from build123d import *

# Parameters (mm, degrees)
F3_D     = 1.1
F5_DEPTH = 11


with BuildPart() as f1:
    # F0 (on Front) → F1 (revolve)
    with BuildSketch(Plane.XZ):
        with BuildLine():
            Line((0, 18), (0, 0))
            Line((0, 0), (22.892781, 0))
            ThreePointArc((22.892781, 0), (24.331991, 1.077301), (23.703917, 2.761768))
            Line((23.703917, 2.761768), (0, 18))
        make_face()
    revolve(axis=Axis((11.44639, 0, 0), (1, 0, 0)))

    # F3 (through all)
    with Locations(Plane(origin=(0, 0, 0), x_dir=(0, 1, 0), z_dir=(-1, 0, 0))):
        with Locations((0, 0)):
            Hole(F3_D / 2)

    # F4 (on Right) → F5 (cut)
    with BuildSketch(Plane.YZ):
        Polygon((-1.6, -8.85), (-1.6, -14.6), (1.6, -14.6), (1.6, -8.85), (1.6, -4.6), (-1.6, -4.6), align=None)
    extrude(amount=F5_DEPTH, mode=Mode.SUBTRACT)


solid = f1.part
Geometry check sheet. Reference: the model listing, model coordinates, mm. A direction names the side the tool comes from. Give positions to 0.01 mm unless a question says otherwise; leave off trailing zeros. Order: outer loops, then holes, each group sorted by start corner. A loop starts at its lowest first (then second) coordinate and runs counter-clockwise, first axis right, second up. Notation, with made-up numbers: (-17.75, 16) - (37.25, 16) arc R20 ccw to (37.25, 46) - close; hole circle Ø9 at (-6, 23). An arc over 180 degrees is marked (long way). Answer as a JSON object with one key per item and string values.
(1) Cross-section at C-C (x = 14.5). Record the cut outline in (y, z), then the cut area to 3 significant figures.
Report:
{"outline": "circle Ø17.36 at (0, 0); hole circle Ø1.1 at (0, 0)", "area": "236 mm^2"}
(2) Draft check along Y on faces 1 (the flat face through (5, 1.6, -10)), 2 (the flat face through (0, 0, 4)), 3 (the conical face through (16.95, 2.72, 6.56)). Enter one of: released by +Y, released by -Y, zero draft, split by the parting line, or undercut.
Report:
{"face 1": "undercut", "face 2": "zero draft", "face 3": "split by the parting line"}
(3) Cross-section at D-D (x = 9). Record the cut outline in (y, z).
Report:
{"outline": "(-1.6, -12.11) - (-1.6, -4.6) - (1.6, -4.6) - (1.6, -12.11) arc R12.21 ccw (long way) to start; hole circle Ø1.1 at (0, 0)"}
(4) Material ranges on line 1 (Z direction, x = 18.5, y = 0); line 2 (Z direction, x = 4, y = 14); line 3 (Z direction, x = 7.25, y = 4.5), recorded low to high.
Report:
{"line 1": "-6.11 to -0.55, 0.55 to 6.11", "line 2": "-6.48 to 6.48", "line 3": "-12.56 to 12.56"}
(5) Tool access check on faces 4 (the flat face through (3, 0, -14.6)), 5 (the flat face through (5, -1.6, -10)), 6 (the flat face through (11, 0, -8)). Record the directions out of +Z, -Z, +X, -X, +Y, -Y that give a thin tool (end or side, any length) a straight path to the whole face; none if there is none.
Report:
{"face 4": "+X, -X", "face 5": "-X", "face 6": "-Z, -X"}
(6) Cross-section at A-A (y = 0). State how many separate pieces and enclosed holes the cut face has, then the cut area to 3 significant figures.
Report:
{"separate pieces": "3", "enclosed holes": "0", "area": "369 mm^2"}
(7) Cross-section at B-B (x = 17.75). Record the cut outline in (y, z), then the cut area to 3 significant figures.
Report:
{"outline": "circle Ø13.18 at (0, 0); hole circle Ø1.1 at (0, 0)", "area": "135 mm^2"}
(8) Depth check by flat-ended pin: pin 1 Ø1 at (x, z) = (3.5, -5) entering from +Y; pin 2 Ø3 at (x, z) = (7.5, -11) entering from -Y; pin 3 Ø5 at (x, z) = (5.5, -12) entering from +Y. Enter the tip coordinate at first touch or a pass-through.
Report:
{"pin 1": "y = 15.31", "pin 2": "y = -9.66", "pin 3": "y = 11.78"}
